Build history of the part. All positions in model axes, mm. Face numbers are marked on the shaded views. A direction names the side the tool comes from. Round coordinates to 2 decimals unless told otherwise and drop trailing zeros. Loops run counter-clockwise (first coordinate to the right, second up) from the corner with the lowest first, then second, coordinate; pieces in that order, holes last. Notation, with made-up numbers: (-0.5, -20.5) - (23.5, -20.5) arc R18 cw to (23.5, 4.5) - close; hole circle Ø9 at (40, 39.25). An arc over 180 degrees is marked (long way). Use a Markdown table: item, result.
Autodesk Inventor part; units mm, degrees
ref_plane "YZ Plane" through (0, 0, 0) normal (1, 0, 0) x (0, 1, 0)
ref_plane "XZ Plane" through (0, 0, 0) normal (0, 1, 0) x (-1, 0, 0)
ref_plane "XY Plane" through (0, 0, 0) normal (0, 0, 1) x (1, 0, 0)
sketch "Sketch1" plane through (0, 0, 0) normal (0, 0, 1) x (1, 0, 0)
  line L0 (0, 0) -> (60, 0)
  line L1 (60, 0) -> (60, 42.4)
  line L2 (60, 42.4) -> (0, 42.4)
  line L3 (0, 42.4) -> (0, 0)
  circle A0 centre (5, 33.4) radius 2.1
  circle A1 centre (55, 33.4) radius 2.1
  circle A2 centre (55, 9) radius 2.1
  circle A3 centre (5, 9) radius 2.1
  circle A4 centre (30, 21.2) radius 5
  circle A5 centre (14.5, 36.7) radius 3
  circle A6 centre (45.5, 36.7) radius 3
  circle A7 centre (45.5, 5.7) radius 3
  circle A8 centre (14.5, 5.7) radius 3
  dimension "d0" = 42.4
  dimension "d1" = 60
  dimension "d2" = 10
  dimension "d3" = 4.2
  dimension "d4" = 24.4
  dimension "d5" = 50
  dimension "d6" = 9
  dimension "d7" = 5
  dimension "d8" = 6
  dimension "d9" = 31
  dimension "d10" = 31
  dimension "d11" = 5.7
  dimension "d12" = 14.5
  dimension "d13" = 30
  dimension "d14" = 21.2
extrude "Extrusion1" add sketch "Sketch1" along normal blind 18
fillet "Fillet1" radius 1 11 edges at (0, 42.4, 9) (60, 42.4, 9) (30, 42.4, 0) (60, 21.2, 18) (30, 0, 18) (0, 21.2, 18) (0, 0, 9) (0, 21.2, 0) (60, 0, 9) (60, 21.2, 0) (30, 0, 0)
fillet "Fillet2" radius 3 3 edges at (30, 42.4, 18) (59.7071, 42.1071, 17.7071) (0.2929, 42.1071, 17.7071)
sketch "Sketch2" plane through (0, 0, 18) normal (0, 0, 1) x (1, 0, 0)
  circle A0 centre (5, 33.4) radius 2.1
  circle A1 centre (55, 33.4) radius 2.1
  circle A2 centre (55, 9) radius 2.1
  circle A3 centre (5, 9) radius 2.1
  circle A4 centre (5, 33.4) radius 4.25
  circle A5 centre (55, 33.4) radius 4.25
  circle A6 centre (55, 9) radius 4.25
  circle A7 centre (5, 9) radius 4.25
  point P0 (0, 0)
  dimension "d19" = 8.5
extrude "Extrusion2" cut sketch "Sketch2" against normal blind 4
sketch "Sketch3" plane through (1, 0, 1) normal (0, -1, 0) x (1, 0, 0)
  line L0 (27, 17) -> (40, 17)
  line L1 (40, 17) -> (40, 7)
  line L2 (40, 7) -> (27, 7)
  line L3 (27, 7) -> (27, 17)
  line L4 (58, 17) -> (0, 17)
  line L5 (59, 0) -> (59, 16)
  point P0 (-1, -1)
  dimension "d22" = 19
  dimension "d23" = 13
  dimension "d24" = 10
extrude "Extrusion3" cut sketch "Sketch3" against normal blind 6
sketch "Sketch4" plane through (1, 0, 1) normal (0, -1, 0) x (1, 0, 0)
  line L0 (27, 7) -> (27, 16)
  circle A0 centre (30.25, 12) radius 1.05
  circle A1 centre (36.75, 12) radius 1.05
  line L1 (27, 17) -> (0, 17)
  point P0 (-1, -1)
  dimension "d27" = 2.1
  dimension "d28" = 5
  dimension "d29" = 6.5
  dimension "d30" = 3.25
extrude "Extrusion4" cut sketch "Sketch4" against normal blind 14
sketch "Sketch5" plane through (0, 0, 18) normal (0, 0, 1) x (1, 0, 0)
  circle A0 centre (30, 21.2) radius 5
  circle A1 centre (30, 21.2) radius 7.1
  point P0 (0, 0)
  dimension "d33" = 14.2
extrude "Extrusion5" cut sketch "Sketch5" against normal blind 15.5
equation "\"d6\" = -0.5 * d4 + 0.5 * d0"
equation "\"d7\" = -0.5 * d5 + 0.5 * d1"
equation "\"d11\" = -0.5 * d10 + 0.5 * d0"
equation "\"d12\" = -0.5 * d9 + 0.5 * d1"
equation "\"d13\" = 0.5 * d1"
equation "\"d14\" = 0.5 * d0"
properties part number "V5 Z Top bearing"
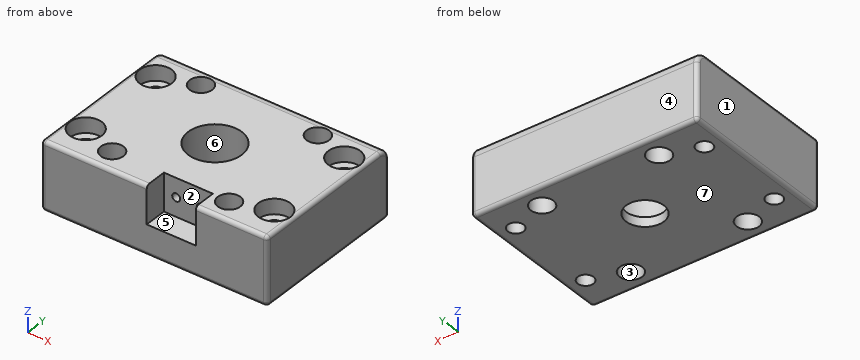
Q1. Cut at D-D, the plane x = 33.5. List the corners of the cut face in (y, z).
Results found:
| item | result |
|---|---|
| outline | (0, 1) arc R1 ccw to (1, 0) - (17.63, 0) - (17.63, 2.5) - (15.02, 2.5) - (15.02, 18) - (6, 18) - (6, 8) - (0, 8) - close; (24.77, 0) - (41.4, 0) arc R1 ccw to (42.4, 1) - (42.4, 15) arc R3 ccw to (39.4, 18) - (27.38, 18) - (27.38, 2.5) - (24.77, 2.5) - close |
Q2. Cut at B-B, the plane y = 21.2. List the corners of the cut face in (x, z).
Results found:
| item | result |
|---|---|
| outline | (0, 1) arc R1 ccw to (1, 0) - (25, 0) - (25, 2.5) - (22.9, 2.5) - (22.9, 18) - (1, 18) arc R1 ccw to (0, 17) - close; (35, 0) - (59, 0) arc R1 ccw to (60, 1) - (60, 17) arc R1 ccw to (59, 18) - (37.1, 18) - (37.1, 2.5) - (35, 2.5) - close |
Q3. Cut at A-A, the plane x = 5. List the corners of the cut face in (y, z).
Results found:
| item | result |
|---|---|
| outline | (0, 1) arc R1 ccw to (1, 0) - (6.9, 0) - (6.9, 14) - (4.75, 14) - (4.75, 18) - (1, 18) arc R1 ccw to (0, 17) - close; (11.1, 0) - (31.3, 0) - (31.3, 14) - (29.15, 14) - (29.15, 18) - (13.25, 18) - (13.25, 14) - (11.1, 14) - close; (35.5, 0) - (41.4, 0) arc R1 ccw to (42.4, 1) - (42.4, 15) arc R3 ccw to (39.4, 18) - (37.65, 18) - (37.65, 14) - (35.5, 14) - close |
Q4. Drop flat-ended pins along their axis: pin 1 (7 mm diameter, centred on x = 45.5, y = 36.7, fed in from -Z); pin 2 (1 mm diameter, centred on x = 38, z = 13, fed in from -Y); pin 3 (1.8 mm diameter, centred on x = 32.5, y = 4, fed in from +Z); pin 4 (7.5 mm diameter, centred on x = 5, y = 9, fed in from +Z). Give the stop position or say it passes through.
Results found:
| item | result |
|---|---|
| pin 1 | stops at z = 0 |
| pin 2 | stops at y = 14 |
| pin 3 | stops at z = 8 |
| pin 4 | stops at z = 14 |
Q5. Which spindle directions (+Z, -Z, +X, -X, +Y, -Y) get a long thin tool onto all of the face, cutting with end or side? Do the marked faces 5, 6 and 7. Say none if no direction does.
Results found:
| item | result |
|---|---|
| face 5 | +Z, -Y |
| face 6 | +Z |
| face 7 | -Z, +X, -X, +Y, -Y |
Q6. Cut at C-C, the plane z = 7.25. Count the separate pieces of the cut face and the enclosed holes in it, plus the area to 3 significant figures.
Results found:
| item | result |
|---|---|
| separate pieces | 1 |
| enclosed holes | 9 |
| area | 2,220 mm2 |
Q7. Pull direction X, two halves, no side cores. Call the marked faces 1, 2, 3 and 4: pulls with the +X half, pulls with the -X half, needs draft (parallel to the pull), parting line crosses it, or undercut.
Results found:
| item | result |
|---|---|
| face 1 | pulls with the -X half |
| face 2 | undercut |
| face 3 | undercut |
| face 4 | needs draft |
Q8. Probe line 1 (X direction, y = 36.7, z = 7.5); line 2 (Y direction, x = 52.5, z = 16); line 3 (X direction, y = 3.5, z = 9). List the from-to ranges inside material, lowest first.
Results found:
| item | result |
|---|---|
| line 1 | x = 0 to 11.5, 17.5 to 42.5, 48.5 to 60 |
| line 2 | y = 0 to 5.56, 12.44 to 29.96, 36.84 to 42.23 |
| line 3 | x = 0 to 12.46, 16.54 to 28, 41 to 43.46, 47.54 to 60 |
